Geometry check sheet. Reference: the model listing, model coordinates, mm. A direction names the side the tool comes from. Round coordinates to 2 decimals unless told otherwise and drop trailing zeros. Order: outer loops, then holes, each group sorted by start corner. A loop starts at its lowest first (then second) coordinate and runs counter-clockwise, first axis right, second up. Notation, with made-up numbers: (69, 29) - (91, 29) arc R14 cw to (91, 40) - close; hole circle Ø1 at (20.25, 52). An arc over 180 degrees is marked (long way). Return JSON: item names as keys, results as strings. Group by question number.
Q1. Sectioned sample at D-D, the plane x = -11. Record the cut outline in (y, z) (3 decimals).
Q2. Draft check along Z on faces 1 (the flat face through (1, 2, 1)), 2 (the flat face through (53, 16, -36.5)), 3 (the flat face through (-57, 15, -1)). Enter one of: pulls with the +Z half, pulls with the -Z half, needs draft (parallel to the pull), parting line crosses it, or undercut.
Q3. Tool access check on faces 4 (the flat face through (-53, 16, -36.5)), 5 (the flat face through (57, 15, 1)), 6 (the cylindrical face through (56, 19.3, 25.5)). Record the directions out of +Z, -Z, +X, -X, +Y, -Y that give a thin tool (end or side, any length) a straight path to the whole face; none if there is none.
Q4. Gauge pin test, flat ends, axial feed: pin 1 Ø3 at (x, z) = (45.5, -36) entering from +Y; pin 2 Ø6 at (x, z) = (21, -1) entering from +Y. Record the tip position at first contact, or that the pin passes through.
Q5. Sectioned sample at A-A, the plane y = 4. Give the number of separate pieces and of enclosed holes in the cut face, then the cut area to 3 significant figures.
Q6. Material ranges on line 1 along Z through (x, y) = (-6, 5.5); line 2 along X through (y, z) = (12.75, -36); line 3 along Z through (x, y) = (-45.5, 7.75), recorded low to high.
Q7. Sectioned sample at B-B, the plane z = -21. Record the cut outline in (x, y), then the cut area to 3 significant figures.
Q8. Sectioned sample at C-C, the plane x = 24.5. Record the cut outline in (y, z) (3 decimals).
Autodesk Inventor part; units mm, degrees
ref_plane "YZ Plane" through (0, 0, 0) normal (1, 0, 0) x (0, 1, 0)
ref_plane "XZ Plane" through (0, 0, 0) normal (0, 1, 0) x (-1, 0, 0)
ref_plane "XY Plane" through (0, 0, 0) normal (0, 0, 1) x (1, 0, 0)
sketch "Sketch1" plane through (0, 0, 0) normal (0, 1, 0) x (-1, 0, 0)
  line L0 (55, -40.5) -> (-55, -40.5)
  line L1 (-55, -40.5) -> (-55, 40.5)
  line L2 (-55, 40.5) -> (55, 40.5)
  line L3 (55, 40.5) -> (55, -40.5)
  line L4 (55, -40.5) -> (-55, 40.5) construction
  line L5 (-55, -40.5) -> (55, 40.5) construction
  line L6 (57, 42.5) -> (-57, 42.5)
  line L7 (-57, 42.5) -> (-57, -42.5)
  line L8 (-57, -42.5) -> (57, -42.5)
  line L9 (57, -42.5) -> (57, 42.5)
  line L10 (57, 42.5) -> (-57, -42.5) construction
  line L11 (-57, 42.5) -> (57, -42.5) construction
  line L12 (50.43, 39.125) -> (-50.43, 39.125)
  line L13 (-50.43, 39.125) -> (-50.43, -39.125)
  line L14 (-50.43, -39.125) -> (50.43, -39.125)
  line L15 (50.43, -39.125) -> (50.43, 39.125)
  line L16 (50.43, 39.125) -> (-50.43, -39.125) construction
  line L17 (-50.43, 39.125) -> (50.43, -39.125) construction
  point P0 (0, 0)
  dimension "d0" = 110
  dimension "d1" = 81
  dimension "d2" = 114
  dimension "d3" = 85
  dimension "d190" = 100.86
  dimension "d191" = 78.25
extrude "Extrusion1" add sketch "Sketch1" along normal blind 30 contours L9 L8 L7 L6
sketch "Sketch2" plane through (0, 0, 0) normal (0, 1, 0) x (-1, 0, 0)
  line L0 (-55, -40.5) -> (-55, 40.5)
  line L1 (55, 40.5) -> (-55, 40.5)
  line L2 (-55, 40.5) -> (-55, -40.5)
  line L3 (-55, -40.5) -> (55, -40.5)
  line L4 (55, -40.5) -> (55, 40.5)
  line L5 (55, 40.5) -> (-55, -40.5) construction
  line L6 (-55, 40.5) -> (55, -40.5) construction
  point P0 (0, 0)
extrude "Extrusion2" add sketch "Sketch2" along normal blind 2
sketch "Sketch3" plane through (0, 0, 0) normal (0, -1, 0) x (1, 0, 0)
  line L0 (44.07, -32.875) -> (-28.43, -32.875)
  line L1 (-28.43, -32.875) -> (-28.43, -7.875)
  line L2 (-28.43, -7.875) -> (44.07, -7.875)
  line L3 (44.07, -7.875) -> (44.07, -32.875)
  line L4 (34.53, 35.725) -> (6.53, 35.725)
  line L5 (6.53, 35.725) -> (6.53, 7.725)
  line L6 (6.53, 7.725) -> (34.53, 7.725)
  line L7 (34.53, 7.725) -> (34.53, 35.725)
  line L8 (-7.03, 11.425) -> (-17.03, 11.425)
  line L9 (-17.03, 11.425) -> (-17.03, 6.425)
  line L10 (-17.03, 6.425) -> (-7.03, 6.425)
  line L11 (-7.03, 6.425) -> (-7.03, 11.425)
  line L12 (50.43, 39.125) -> (-50.43, 39.125)
  line L13 (-50.43, 39.125) -> (-50.43, -39.125)
  line L14 (-50.43, -39.125) -> (50.43, -39.125)
  line L15 (50.43, -39.125) -> (50.43, 39.125)
  line L16 (50.43, 39.125) -> (-50.43, -39.125) construction
  line L17 (-50.43, 39.125) -> (50.43, -39.125) construction
  line L18 (-30.4304, 18.225) -> (-37.4304, 18.225)
  line L19 (-37.4304, 18.225) -> (-37.4304, 11.225)
  line L20 (-37.4304, 11.225) -> (-30.4304, 11.225)
  line L21 (-30.4304, 11.225) -> (-30.4304, 18.225)
  line L22 (-30.4304, 18.225) -> (-37.4304, 11.225) construction
  line L23 (-37.4304, 18.225) -> (-30.4304, 11.225) construction
  line L24 (-30.4304, 33.4598) -> (-37.4304, 33.4598)
  line L25 (-37.4304, 33.4598) -> (-37.4304, 26.4598)
  line L26 (-37.4304, 26.4598) -> (-30.4304, 26.4598)
  line L27 (-30.4304, 26.4598) -> (-30.4304, 33.4598)
  line L28 (-30.4304, 33.4598) -> (-37.4304, 26.4598) construction
  line L29 (-37.4304, 33.4598) -> (-30.4304, 26.4598) construction
  line L30 (-23.8133, 25.9138) -> (-30.8133, 25.9138)
  line L31 (-30.8133, 25.9138) -> (-30.8133, 18.9138)
  line L32 (-30.8133, 18.9138) -> (-23.8133, 18.9138)
  line L33 (-23.8133, 18.9138) -> (-23.8133, 25.9138)
  line L34 (-23.8133, 25.9138) -> (-30.8133, 18.9138) construction
  line L35 (-30.8133, 25.9138) -> (-23.8133, 18.9138) construction
  line L36 (-36.8875, 25.9138) -> (-43.8875, 25.9138)
  line L37 (-43.8875, 25.9138) -> (-43.8875, 18.9138)
  line L38 (-43.8875, 18.9138) -> (-36.8875, 18.9138)
  line L39 (-36.8875, 18.9138) -> (-36.8875, 25.9138)
  line L40 (-36.8875, 25.9138) -> (-43.8875, 18.9138) construction
  line L41 (-43.8875, 25.9138) -> (-36.8875, 18.9138) construction
  line L42 (-50.43, 39.125) -> (50.4731, 39.0489) construction
  line L43 (50.4731, 39.0489) -> (50.4141, -39.1891) construction
  line L44 (50.4141, -39.1891) -> (-50.489, -39.113) construction
  line L45 (-50.489, -39.113) -> (-50.43, 39.125) construction
  line L46 (17.9042, 35.3523) -> (15.6181, 35.3523)
  line L47 (47.7465, 12.6947) -> (44.5311, 12.6947)
  line L48 (46.7465, 20.4524) -> (43.1682, 20.4524)
  line L49 (-57, 42.5) -> (57, 42.5)
  line L50 (-44.8275, -6.6468) -> (-48.1514, -6.6468)
  line L51 (-48.1514, -6.6468) -> (-48.1514, 1.9287)
  line L52 (-48.1514, 1.9287) -> (-44.8275, 1.9287)
  line L53 (-44.8275, 1.9287) -> (-44.8275, -6.6468)
  line L54 (-44.8275, 4.375) -> (-48.1514, 4.375)
  line L55 (-48.1514, 4.375) -> (-48.1514, 10.225)
  line L56 (-48.1514, 10.225) -> (-44.8275, 10.225)
  line L57 (-44.8275, 10.225) -> (-44.8275, 4.375)
  point P0 (0, 0)
  point P1 (-33.9304, 14.725)
  point P2 (-33.9304, 29.9598)
  point P3 (-27.3133, 22.4138)
  point P4 (-40.3875, 22.4138)
  point P5 (46.1388, 12.6947)
  dimension "d8" = 72.5
  dimension "d9" = 25
  dimension "d18" = 28
  dimension "d19" = 28
  dimension "d20" = 10
  dimension "d21" = 5
  dimension "d22" = 100.86
  dimension "d23" = 78.25
  dimension "d31" = 3.4
  dimension "d32" = 15.9
  dimension "d33" = 22
  dimension "d35" = 33.4
  dimension "d36" = 27.7
  dimension "d45" = 7
  dimension "d46" = 7
  dimension "d47" = 7
  dimension "d48" = 7
  dimension "d135" = 7
  dimension "d136" = 7
  dimension "d137" = 7
  dimension "d138" = 7
  dimension "d203" = 47
  dimension "d580" = 3.7727
  dimension "d585" = 22.0476
extrude "Extrusion3" cut sketch "Sketch3" against normal blind 30 contours L0 L1 L2 L3 | L7 L6 L5 L4 | L11 L10 L9 L8 | L21 L20 L19 L18 | L27 L26 L25 L24 | L33 L32 L31 L30 | L39 L38 L37 L36 | L50 L51 L52 L53 | L54 L55 L56 L57
sketch "Sketch4" plane through (0, 2, 0) normal (0, 1, 0) x (1, 0, 0)
  circle A0 centre (-45.13, -34.025) radius 1.25
  line L0 (55, -40.5) -> (-55, -40.5)
  line L1 (-55, -40.5) -> (-55, 40.5)
  circle A1 centre (-42.23, 34.175) radius 1.25
  line L2 (-55, 40.5) -> (55, 40.5)
  circle A2 centre (45.31, -34.725) radius 1.25
  line L3 (55, 40.5) -> (55, -40.5)
  line L4 (-50.43, -39.125) -> (50.43, -39.125)
  line L5 (50.43, -39.125) -> (50.43, 39.125)
  line L6 (50.43, 39.125) -> (-50.43, 39.125)
  line L7 (-50.43, 39.125) -> (-50.43, -39.125)
  line L8 (-50.43, -39.125) -> (50.43, 39.125) construction
  line L9 (50.43, -39.125) -> (-50.43, 39.125) construction
  circle A3 centre (-30.23, 36.375) radius 1.25
  circle A4 centre (45.87, 36.375) radius 1.25
  circle A5 centre (-30.23, 5.375) radius 1.25
  circle A6 centre (45.87, 5.375) radius 1.25
  line L10 (-28.43, 7.875) -> (-28.43, 32.875)
  line L11 (44.07, 32.875) -> (44.07, 7.875)
  line L12 (-28.43, 32.875) -> (44.07, 32.875)
  line L13 (44.07, 7.875) -> (-28.43, 7.875)
  line L14 (-50.43, 39.125) -> (50.4734, 39.0562) construction
  line L15 (50.4734, 39.0562) -> (50.42, -39.1821) construction
  line L16 (50.42, -39.1821) -> (-50.4834, -39.1133) construction
  line L17 (-50.4834, -39.1133) -> (-50.43, 39.125) construction
  point P0 (0, 0)
  dimension "d181" = 2.5
  dimension "d184" = 2.5
  dimension "d187" = 2.5
  dimension "d192" = 100.86
  dimension "d193" = 78.25
  dimension "d194" = 8.2
  dimension "d195" = 4.95
  dimension "d196" = 5.3
  dimension "d197" = 5.1
  dimension "d198" = 5.12
  dimension "d199" = 4.4
  dimension "d204" = 2.5
  dimension "d205" = 2.5
  dimension "d206" = 2.5
  dimension "d207" = 2.5
  dimension "d209" = 1.8
  dimension "d211" = 1.8
  dimension "d212" = 1.8
  dimension "d213" = 1.8
  dimension "d214" = 3.5
  dimension "d215" = 3.5
  dimension "d216" = 2.5
  dimension "d217" = 2.5
extrude "Extrusion4" add sketch "Sketch4" along normal blind 6 contours A0 | A1 | A2 | A3 | A4 | A5 | A6
sketch "Sketch5" plane through (0, 2, 0) normal (0, 1, 0) x (1, 0, 0)
  line L0 (50.43, 39.125) -> (-50.43, 39.125)
  line L1 (-50.43, 39.125) -> (-50.43, -39.125)
  line L2 (-50.43, -39.125) -> (50.43, -39.125)
  line L3 (50.43, -39.125) -> (50.43, 39.125)
  line L4 (50.43, 39.125) -> (-50.43, -39.125) construction
  line L5 (-50.43, 39.125) -> (50.43, -39.125) construction
  point P0 (0, 0)
  dimension "d352" = 78.25
  dimension "d353" = 100.86
sketch "Sketch6" plane through (0, 2, 0) normal (0, 1, 0) x (1, 0, 0)
  line L0 (55, -40.5) -> (-55, -40.5)
  line L1 (55, -40.5) -> (51, -40.5)
  line L2 (51, -40.5) -> (51, -36.5)
  line L3 (51, -36.5) -> (55, -36.5)
  line L4 (55, -36.5) -> (55, -40.5)
  line L5 (-55, 40.5) -> (55, 40.5)
  line L6 (55, 40.5) -> (51, 40.5)
  line L7 (51, 40.5) -> (51, 36.5)
  line L8 (51, 36.5) -> (55, 36.5)
  line L9 (55, 36.5) -> (55, 40.5)
  line L10 (-54.9902, -40.5) -> (-50.9902, -40.5)
  line L11 (-50.9902, -40.5) -> (-50.9902, -36.5)
  line L12 (-50.9902, -36.5) -> (-54.9902, -36.5)
  line L13 (-54.9902, -36.5) -> (-55, -36.5)
  line L14 (55, -40.5) -> (-55, -40.5)
  line L15 (-50.9902, -40.5) -> (-55, -40.5)
  line L16 (-55, -40.5) -> (-55, -36.5)
  line L17 (-55, 40.5) -> (55, 40.5)
  line L18 (-50.424, 39.0879) -> (50.4561, 39.0879) construction
  line L19 (50.4561, 39.0879) -> (50.4561, -39.1323) construction
  line L20 (50.4561, -39.1323) -> (-50.424, -39.1323) construction
  line L21 (-50.424, -39.1323) -> (-50.424, 39.0879) construction
  line L22 (-49.2051, 39.0879) -> (-45.6234, 39.0879)
  line L23 (-48.1397, 6.687) -> (-44.6458, 6.687)
  line L24 (-48.2072, -10.3595) -> (-44.6458, -10.3595)
  line L25 (-55, 40.5) -> (-51, 40.5)
  line L26 (-51, 40.5) -> (-51, 36.5)
  line L27 (-51, 36.5) -> (-55, 36.5)
  line L28 (-55, 36.5) -> (-55, 40.5)
  line L29 (-51, 40.5) -> (51, 40.5)
  line L30 (57, 42.5) -> (-57, 42.5)
  line L31 (55, 36.5) -> (55, -36.5)
  line L32 (51, -40.5) -> (-50.9902, -40.5)
  line L33 (-55, -36.5) -> (-55, 36.5)
  line L34 (55, 40.5) -> (55, -40.5)
  line L35 (55, 40.5) -> (55, -40.5)
  line L36 (55, 40.5) -> (55, -40.5)
  point P0 (0, 0)
  dimension "d443" = 4
  dimension "d444" = 4
  dimension "d445" = 4
  dimension "d446" = 4
  dimension "d447" = 4
  dimension "d448" = 4
  dimension "d564" = 30.1405
  dimension "d591" = 4
  dimension "d592" = 4
  dimension "d599" = 110
  dimension "d600" = 81
extrude "Extrusion5" add sketch "Sketch6" along normal up to surface (28 mm away) contours L0 L2 L3 L4 | L0 L16 L13 L12 L11 | L8 L7 L5 L9 | L26 L27 L28 L5
sketch "Sketch8" plane through (57, 0, 42.5) normal (1, 0, 0) x (0, 0, -1)
  line L0 (28, 23.25) -> (28, 15.25) construction
  line L1 (28, 23.25) -> (36, 23.25) construction
  line L2 (28, 15.25) -> (21, 15.25)
  line L3 (21, 15.25) -> (22.6917, 15.25)
  line L4 (28, 23.25) -> (21, 23.25)
  arc A0 (21, 23.25) -> (21, 15.25) centre (21, 19.25) ccw
  arc A1 (28, 15.25) -> (28, 23.25) centre (28, 19.25) ccw
  line L5 (0, 30) -> (85, 30)
  line L6 (0, 0) -> (0, 30)
  line L7 (0, 0) -> (85, 0)
  line L8 (24.5, 23.25) -> (24.5, 15.25) construction
  point P0 (42.5, 0)
  point P1 (0, 15)
  point P2 (17, 19.25)
  point P3 (24.5, 19.25)
  dimension "d573" = 90
  dimension "d574" = 7
  dimension "d609" = 24.5
  dimension "d610" = 8
  dimension "d611" = 10.75
extrude "Extrusion9" cut sketch "Sketch8" against normal blind 3
properties part number "plant watner 2.0 case"
Reply:
{
 "1": {"outline": "(0, -42.5) - (30, -42.5) - (30, -40.5) - (2, -40.5) - (2, -32.875) - (0, -32.875) - close; (0, -7.875) - (2, -7.875) - (2, 6.425) - (0, 6.425) - close; (0, 11.425) - (2, 11.425) - (2, 40.5) - (30, 40.5) - (30, 42.5) - (0, 42.5) - close"},
 "2": {"face 1": "undercut", "face 2": "undercut", "face 3": "needs draft"},
 "3": {"face 4": "+Y", "face 5": "+Z, -Z, +X, +Y, -Y", "face 6": "+X"},
 "4": {"pin 1": "y = 8", "pin 2": "y = 2"},
 "5": {"separate pieces": "8", "enclosed holes": "1", "area": "878 mm^2"},
 "6": {"line 1": "-42.5 to -40.5, 40.5 to 42.5", "line 2": "-57 to -55, 55 to 57", "line 3": "-42.5 to -40.5, 32.83 to 35.22, 40.5 to 42.5"},
 "7": {"outline": "(-57, 0) - (-28.43, 0) - (-28.43, 2) - (-55, 2) - (-55, 30) - (-57, 30) - close; (44.07, 0) - (57, 0) - (57, 30) - (55, 30) - (55, 2) - (44.07, 2) - close", "area": "195 mm^2"},
 "8": {"outline": "(0, -42.5) - (30, -42.5) - (30, -40.5) - (2, -40.5) - (2, -32.875) - (0, -32.875) - close; (0, -7.875) - (2, -7.875) - (2, 7.725) - (0, 7.725) - close; (0, 35.725) - (2, 35.725) - (2, 40.5) - (30, 40.5) - (30, 42.5) - (0, 42.5) - close"}
}
